Geometry: final body of the model. Coordinates: model frame, mm. Coordinates: 2 decimals unless noted, no trailing zeros. Loops run counter-clockwise (first coordinate to the right, second up) from the corner with the lowest first, then second, coordinate; pieces in that order, holes last. Notation, with made-up numbers: (57, 74.25) - (62, 74.25) arc R11 cw to (62, 83.25) - close; hole circle Ø1 at (63, -14.5). An arc over 180 degrees is marked (long way). Answer in a Markdown table with one row per item.
from build123d import *

# Parameters (mm, degrees)
SKETCH_1_W      = 31.8
SKETCH_1_H      = 20.3
EXTRUDE_1_DEPTH = 10.2
FILLET_2_R      = 1
FILLET_1_R      = 3
SKETCH_2_R      = 0.25
EXTRUDE_2_DEPTH = 3.05


with BuildPart() as part:
    # Эскиз1 → Бобышка-Вытянуть1 (new body)
    with BuildSketch(Plane.XY):
        Rectangle(SKETCH_1_W, SKETCH_1_H)
    extrude(amount=EXTRUDE_1_DEPTH)

    # Скругление2
    fillet_2_edges = [part.edges().sort_by_distance(p)[0] for p in [
        (-15.9, 0, 10.2),
        (0, -10.15, 10.2),
        (15.9, 0, 10.2),
        (0, -10.15, 0),
        (-15.9, 0, 0),
        (0, 10.15, 0),
        (15.9, 0, 0),
        (0, 10.15, 10.2),
    ]]
    fillet(fillet_2_edges, radius=FILLET_2_R)

    # Скругление1
    # the kernel refuses this fillet: 3 mm, written as the material it takes off along each edge
    with BuildSketch(Plane(origin=(12.9, -7.15, 0), x_dir=(1, 0, 0), z_dir=(0, 1, 0))) as fillet_1_piece_1:
        with BuildLine():
            CenterArc((2, -1), 1, 0, 90)
            Line((3, -1), (3, 0))
            Line((3, 0), (2, 0))
        make_face()
    revolve(axis=Axis((12.9, -7.15, 0), (0, 0, -1)), revolution_arc=90, mode=Mode.SUBTRACT)
    with BuildSketch(Plane(origin=(-12.9, -7.15, 0), x_dir=(0, -1, 0), z_dir=(1, 0, 0))) as fillet_1_piece_2:
        with BuildLine():
            CenterArc((2, -1), 1, 0, 90)
            Line((3, -1), (3, 0))
            Line((3, 0), (2, 0))
        make_face()
    revolve(axis=Axis((-12.9, -7.15, 0), (0, 0, -1)), revolution_arc=90, mode=Mode.SUBTRACT)
    with BuildSketch(Plane(origin=(12.9, 7.15, 0), x_dir=(0, 1, 0), z_dir=(-1, 0, 0))) as fillet_1_piece_3:
        with BuildLine():
            CenterArc((2, -1), 1, 0, 90)
            Line((3, -1), (3, 0))
            Line((3, 0), (2, 0))
        make_face()
    revolve(axis=Axis((12.9, 7.15, 0), (0, 0, -1)), revolution_arc=90, mode=Mode.SUBTRACT)
    with BuildSketch(Plane(origin=(-12.9, 7.15, 0), x_dir=(-1, 0, 0), z_dir=(0, -1, 0))) as fillet_1_piece_4:
        with BuildLine():
            CenterArc((2, -1), 1, 0, 90)
            Line((3, -1), (3, 0))
            Line((3, 0), (2, 0))
        make_face()
    revolve(axis=Axis((-12.9, 7.15, 0), (0, 0, -1)), revolution_arc=90, mode=Mode.SUBTRACT)
    with BuildSketch(Plane(origin=(12.9, -7.15, 10.2), x_dir=(0, -1, 0), z_dir=(-1, 0, 0))) as fillet_1_piece_5:
        with BuildLine():
            CenterArc((2, -1), 1, 0, 90)
            Line((3, -1), (3, 0))
            Line((3, 0), (2, 0))
        make_face()
    revolve(axis=Axis((12.9, -7.15, 10.2), (0, 0, 1)), revolution_arc=90, mode=Mode.SUBTRACT)
    with BuildSketch(Plane(origin=(-12.9, -7.15, 10.2), x_dir=(-1, 0, 0), z_dir=(0, 1, 0))) as fillet_1_piece_6:
        with BuildLine():
            CenterArc((2, -1), 1, 0, 90)
            Line((3, -1), (3, 0))
            Line((3, 0), (2, 0))
        make_face()
    revolve(axis=Axis((-12.9, -7.15, 10.2), (0, 0, 1)), revolution_arc=90, mode=Mode.SUBTRACT)
    with BuildSketch(Plane(origin=(12.9, 7.15, 10.2), x_dir=(1, 0, 0), z_dir=(0, -1, 0))) as fillet_1_piece_7:
        with BuildLine():
            CenterArc((2, -1), 1, 0, 90)
            Line((3, -1), (3, 0))
            Line((3, 0), (2, 0))
        make_face()
    revolve(axis=Axis((12.9, 7.15, 10.2), (0, 0, 1)), revolution_arc=90, mode=Mode.SUBTRACT)
    with BuildSketch(Plane(origin=(-12.9, 7.15, 10.2), x_dir=(0, 1, 0), z_dir=(1, 0, 0))) as fillet_1_piece_8:
        with BuildLine():
            CenterArc((2, -1), 1, 0, 90)
            Line((3, -1), (3, 0))
            Line((3, 0), (2, 0))
        make_face()
    revolve(axis=Axis((-12.9, 7.15, 10.2), (0, 0, 1)), revolution_arc=90, mode=Mode.SUBTRACT)
    with BuildSketch(Plane(origin=(-15.9, 10.15, 0), x_dir=(0, -1, 0), z_dir=(0, 0, 1)), Plane(origin=(-15.9, -10.15, 0), x_dir=(1, 0, 0), z_dir=(0, 0, 1))) as fillet_1_piece_9:
        with BuildLine():
            CenterArc((FILLET_1_R, FILLET_1_R), FILLET_1_R, 180, 90)
            Line((0, FILLET_1_R), (0, 0))
            Line((0, 0), (FILLET_1_R, 0))
        make_face()
    extrude(amount=10.2, mode=Mode.SUBTRACT)
    with BuildSketch(Plane(origin=(15.9, 10.15, 0), x_dir=(0, -1, 0), z_dir=(0, 0, 1)), Plane(origin=(15.9, -10.15, 0), x_dir=(-1, 0, 0), z_dir=(0, 0, 1))) as fillet_1_piece_10:
        with BuildLine():
            CenterArc((FILLET_1_R, -FILLET_1_R), FILLET_1_R, 90, 90)
            Line((0, -FILLET_1_R), (0, 0))
            Line((0, 0), (FILLET_1_R, 0))
        make_face()
    extrude(amount=10.2, mode=Mode.SUBTRACT)

    # Эскиз2 → Бобышка-Вытянуть2 (add)
    with BuildSketch(Plane(origin=(0, 0, 0), x_dir=(-1, 0, 0), z_dir=(0, 0, -1))):
        with Locations((11.45, 7.62)):
            Circle(SKETCH_2_R)
        with Locations((6.37, 7.62)):
            Circle(SKETCH_2_R)
        with Locations((-8.91, 7.62)):
            Circle(SKETCH_2_R)
        with Locations((-11.45, 7.62)):
            Circle(SKETCH_2_R)
        with Locations((-11.45, -7.62)):
            Circle(SKETCH_2_R)
        with Locations((-8.91, -7.62)):
            Circle(SKETCH_2_R)
        with Locations((6.37, -7.62)):
            Circle(SKETCH_2_R)
        with Locations((11.45, -7.62)):
            Circle(SKETCH_2_R)
    extrude(amount=EXTRUDE_2_DEPTH)


solid = part.part
(1) Cut plane B-B on y = 5.25. Output: boundary loops of the cut face in (x, z).
Verdict:
| item | result |
|---|---|
| outline | (-15.9, 1) arc R1 ccw to (-14.9, 0) - (14.9, 0) arc R1 ccw to (15.9, 1) - (15.9, 9.2) arc R1 ccw to (14.9, 10.2) - (-14.9, 10.2) arc R1 ccw to (-15.9, 9.2) - close |
(2) First-contact query: pin 1 Ø2 at (x, y) = (8, 0) entering from -Z. Flat tip, straight axial feed; report the tip coordinate or a pass-through.
Verdict:
| item | result |
|---|---|
| pin 1 | stops at z = 0 |
(3) Cut plane A-A on x = -3.5. Output: boundary loops of the cut face in (y, z), then the cut area to 3 significant figures.
Verdict:
| item | result |
|---|---|
| outline | (-10.15, 1) arc R1 ccw to (-9.15, 0) - (9.15, 0) arc R1 ccw to (10.15, 1) - (10.15, 9.2) arc R1 ccw to (9.15, 10.2) - (-9.15, 10.2) arc R1 ccw to (-10.15, 9.2) - close |
| area | 206 mm² |
(4) Ray query, probe 1 along Z at (x, y) = (-12, -0.25); probe 2 along X at (y, z) = (-7.25, 7); probe 3 along Y at (x, z) = (-14, 6.5). Return the intervals inside material, ascending.
Verdict:
| item | result |
|---|---|
| probe 1 | z = 0 to 10.2 |
| probe 2 | x = -15.9 to 15.9 |
| probe 3 | y = -9.94 to 9.94 |
